Here's how the part is built. I have some questions about the finished solid (model axes, mm). Round coordinates to 2 decimals unless told otherwise and drop trailing zeros. Order: outer loops, then holes, each group sorted by start corner. A loop starts at its lowest first (then second) coordinate and runs counter-clockwise, first axis right, second up. Notation, with made-up numbers: (-31.5, 20.5) - (-23.5, 20.5) arc R11 ccw to (-23.5, 24.5) - close; hole circle Ø10 at (11.5, 32.5). An arc over 180 degrees is marked (long way). Answer as a JSON object with one key per item and string values.
```python
from build123d import *

# Parameters (mm, degrees)
SKETCH1_W           = 139
SKETCH1_H           = 52
SKETCH1_R           = 3.1
SKETCH1_R_2         = 1.6
SKETCH1_R_3         = 3.75
SKETCH1_W_2         = 3.2
SKETCH1_H_2         = 1.9
SKETCH1_W_3         = 1.2
SKETCH1_H_3         = 2.7
SKETCH1_W_4         = 2.7
SKETCH1_H_4         = 1.2
BOSS_EXTRUDE1_DEPTH = 3
BOSS_EXTRUDE2_DEPTH = 1


with BuildPart() as part:
    # Sketch1 → Boss-Extrude1 (new body)
    with BuildSketch(Plane.XY):
        with Locations((69.5, 26)):
            Rectangle(SKETCH1_W, SKETCH1_H)
        with Locations((22.634375474, 42.047579972)):
            Circle(SKETCH1_R, mode=Mode.SUBTRACT)
        with Locations((4, 38)):
            Circle(SKETCH1_R_2, mode=Mode.SUBTRACT)
        with Locations((135, 38)):
            Circle(SKETCH1_R_2, mode=Mode.SUBTRACT)
        with Locations((135, 16)):
            Circle(SKETCH1_R_2, mode=Mode.SUBTRACT)
        with Locations((4, 16)):
            Circle(SKETCH1_R_2, mode=Mode.SUBTRACT)
        with Locations((14.866068747, 28)):
            Circle(SKETCH1_R_2, mode=Mode.SUBTRACT)
        with Locations((124, 28.922858178)):
            Circle(SKETCH1_R_2, mode=Mode.SUBTRACT)
        with Locations((58.031961536, 17.043942087)):
            Circle(SKETCH1_R_3, mode=Mode.SUBTRACT)
        with Locations((45.857489394, 42.12137557)):
            Circle(SKETCH1_R, mode=Mode.SUBTRACT)
        with Locations((113.702920713, 17.043942087)):
            Circle(SKETCH1_R, mode=Mode.SUBTRACT)
        with Locations((58.031961536, 9.343942087)):
            Rectangle(SKETCH1_W_2, SKETCH1_H_2, mode=Mode.SUBTRACT)
        with Locations((28.634375474, 42.047579972)):
            Rectangle(SKETCH1_W_3, SKETCH1_H_3, mode=Mode.SUBTRACT)
        with BuildLine():
            Line((88.076124719, 14.093942087), (92.202866775, 14.093942087))
            ThreePointArc((92.202866775, 14.093942087), (93.739495747, 17.043942087), (92.202866775, 19.993942087))
            Line((92.202866775, 19.993942087), (88.076124719, 19.993942087))
            ThreePointArc((88.076124719, 19.993942087), (86.539495747, 17.043942087), (88.076124719, 14.093942087))
        make_face(mode=Mode.SUBTRACT)
        with Locations((45.857489394, 36.12137557)):
            Rectangle(SKETCH1_W_4, SKETCH1_H_4, mode=Mode.SUBTRACT)
        with BuildLine():
            Line((28.564994968, 14.093942087), (32.691737024, 14.093942087))
            ThreePointArc((32.691737024, 14.093942087), (34.228365996, 17.043942087), (32.691737024, 19.993942087))
            Line((32.691737024, 19.993942087), (28.564994968, 19.993942087))
            ThreePointArc((28.564994968, 19.993942087), (27.028365996, 17.043942087), (28.564994968, 14.093942087))
        make_face(mode=Mode.SUBTRACT)
        with Locations((119.702920713, 17.043942087)):
            Rectangle(SKETCH1_W_3, SKETCH1_H_3, mode=Mode.SUBTRACT)
    extrude(amount=BOSS_EXTRUDE1_DEPTH)

    # Sketch2 → Boss-Extrude2 (add)
    with BuildSketch(Plane.XY.offset(3)):
        with BuildLine():
            Line((111.153182821, 37.289690551), (112.17756564, 38.314073369))
            ThreePointArc((112.17756564, 38.314073369), (112.884672421, 38.314073369), (112.884672421, 37.606966588))
            Line((112.884672421, 37.606966588), (111.152789219, 35.875083385))
            ThreePointArc((111.152789219, 35.875083385), (100.552285062, 40.48168601), (89.951780905, 35.875083385))
            Line((89.951780905, 35.875083385), (88.219897703, 37.606966588))
            ThreePointArc((88.219897703, 37.606966588), (88.219897703, 38.314073369), (88.927004484, 38.314073369))
            Line((88.927004484, 38.314073369), (89.951387302, 37.289690551))
            ThreePointArc((89.951387302, 37.289690551), (91.441613651, 38.521449423), (93.073591221, 39.558104478))
            Line((93.073591221, 39.558104478), (92.415896966, 40.848902132))
            ThreePointArc((92.415896966, 40.848902132), (92.634404978, 41.521400644), (93.30690349, 41.302892632))
            Line((93.30690349, 41.302892632), (93.964597745, 40.012094978))
            ThreePointArc((93.964597745, 40.012094978), (95.762521649, 40.723062012), (97.63496858, 41.204670755))
            Line((97.63496858, 41.204670755), (97.408342585, 42.635530977))
            ThreePointArc((97.408342585, 42.635530977), (97.823969523, 43.20759238), (98.396030925, 42.791965442))
            Line((98.396030925, 42.791965442), (98.622656921, 41.36110522))
            ThreePointArc((98.622656921, 41.36110522), (100.552285062, 41.48168601), (102.481913203, 41.36110522))
            Line((102.481913203, 41.36110522), (102.708539199, 42.791965442))
            ThreePointArc((102.708539199, 42.791965442), (103.280600601, 43.20759238), (103.696227539, 42.635530977))
            Line((103.696227539, 42.635530977), (103.469601544, 41.204670755))
            ThreePointArc((103.469601544, 41.204670755), (105.342048475, 40.723062012), (107.139972379, 40.012094978))
            Line((107.139972379, 40.012094978), (107.797666634, 41.302892632))
            ThreePointArc((107.797666634, 41.302892632), (108.470165146, 41.521400644), (108.688673158, 40.848902132))
            Line((108.688673158, 40.848902132), (108.030978903, 39.558104478))
            ThreePointArc((108.030978903, 39.558104478), (109.662956473, 38.521449423), (111.153182821, 37.289690551))
        make_face()
    extrude(amount=BOSS_EXTRUDE2_DEPTH)


solid = part.part
```
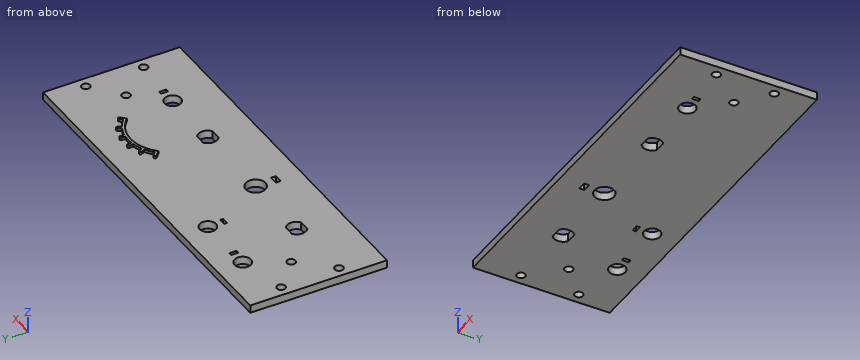
1. For P1, Ø10, axis at x = 118.5, y = 42.5, coming from the +Z side; P2, Ø2.5, axis at x = 124, y = 28.92, coming from the -Z side, each with a flat end and sliding along its axis, tell me the tip position at first contact or that it passes through.
Responses:
{"P1": "z = 3", "P2": "through"}
2. Imagine slicing it at B-B (x = 23.5). List the corners of the cut face in (y, z) for me.
Responses:
{"outline": "(0, 0) - (39.07, 0) - (39.07, 3) - (0, 3) - close; (45.02, 0) - (52, 0) - (52, 3) - (45.02, 3) - close"}
3. Imagine slicing it at A-A (x = 124). List the corners of the cut face in (y, z) for me, plus the area to 3 significant figures.
Responses:
{"outline": "(0, 0) - (27.32, 0) - (27.32, 3) - (0, 3) - close; (30.52, 0) - (52, 0) - (52, 3) - (30.52, 3) - close", "area": "146 mm2"}
4. Imagine slicing it at C-C (y = 24.5). List the corners of the cut face in (x, z) for me, plus the area to 3 significant figures.
Responses:
{"outline": "(0, 0) - (139, 0) - (139, 3) - (0, 3) - close", "area": "417 mm2"}
5. If I drill on L1, parallel to Y at x = 4, z = 2.05; L2, parallel to Y at x = 113.5, z = 0.6; L3, parallel to X at y = 40, z = 1.15, over which ranges is the centre line in solid material (lowest first)? Write a range as [from, to].
Responses:
{"L1": "[0, 14.4], [17.6, 36.4], [39.6, 52]", "L2": "[0, 13.95], [20.14, 52]", "L3": "[0, 20.31], [24.96, 43.6], [48.12, 139]"}
6. Imagine slicing it at D-D (z = 1.95). Give the number of separate pieces and of enclosed holes in the cut face, plus the area to 3 significant figures.
Responses:
{"separate pieces": "1", "enclosed holes": "16", "area": "6,960 mm2"}
